Read the model definition and answer for the solid it produces. Units are mm, in the model's axes. A direction names the side the tool comes from. Coordinates: 2 decimals unless noted, no trailing zeros. Loops run counter-clockwise (first coordinate to the right, second up) from the corner with the lowest first, then second, coordinate; pieces in that order, holes last. Notation, with made-up numbers: M 49,42 L 75,42 A27 cw 75,61 Z; hole C -1,-13 d8. An arc over 180 degrees is marked long. One line per item, written item: value. Start each with the question number.
```python
from build123d import *

# Parameters (mm, degrees)
SKETCH_1_R      = 1.25
EXTRUDE_1_DEPTH = 1.6


with BuildPart() as part:
    # Эскиз1 → Бобышка-Вытянуть1 (new body)
    with BuildSketch(Plane(origin=(0, 0, 0), x_dir=(0, 0, -1), z_dir=(1, 0, 0))):
        with BuildLine():
            Line((2.714158993, 32.8544628), (3.027276679, 29.368497035))
            Line((3.027276679, 29.368497035), (-8.924605944, 28.294950683))
            Line((-8.924605944, 28.294950683), (-9.23772363, 31.780916448))
            ThreePointArc((-9.23772363, 31.780916448), (-9.009264175, 32.511390756), (-8.331195608, 32.866368862))
            Line((-8.331195608, 32.866368862), (-4.596232288, 33.201852097))
            Line((-4.596232288, 33.201852097), (-4.417307896, 31.20987166))
            ThreePointArc((-4.417307896, 31.20987166), (-3.991334168, 30.39618938), (-3.114764999, 30.122038033))
            Line((-3.114764999, 30.122038033), (-3.015165977, 30.130984253))
            ThreePointArc((-3.015165977, 30.130984253), (-2.201483696, 30.55695798), (-1.92733235, 31.43352715))
            Line((-1.92733235, 31.43352715), (-2.106256742, 33.425507587))
            Line((-2.106256742, 33.425507587), (1.628706578, 33.760990822))
            ThreePointArc((1.628706578, 33.760990822), (2.359180886, 33.532531367), (2.714158993, 32.8544628))
        make_face()
        with Locations((-6.635920339, 30.759584164)):
            Circle(SKETCH_1_R, mode=Mode.SUBTRACT)
        with Locations((0.336011191, 31.385819536)):
            Circle(SKETCH_1_R, mode=Mode.SUBTRACT)
    extrude(amount=EXTRUDE_1_DEPTH)


solid = part.part
```
1) Section C-C (y = 32.2) is taken. Determine the outline of the cut face in (x, z).
2) Section B-B (z = 0.25) is taken. Determine the outline of the cut face in (x, y), then the cut area to 3 significant figures.
3) Section A-A (y = 33.05) is taken. Determine the outline of the cut face in (x, z), then the cut area to 3 significant figures.
4) A flat-ended cylindrical pin translates along its axis: pin 1 (1.5 mm diameter, centred on y = 31.39, z = -0.34, fed in from +X). Find the tip coordinate at first contact, or state that the pin passes through.
5) A tool of negligible diameter and unlimited length cuts with its end or side. For faces 1 (the face through (0.789, 32.416, 2.016)), 2 (the face through (0.79, 32.22, 4.51)), 3 (the face through (0, 29.9, 3)), from which of +Z, -Z, +X, -X, +Y, -Y can it reach the whole face along a straight path? Write none if from no direction.
6) For a pull along Y with two mould halves and no side action, classify faces 4 (the face through (0.79, 28.84, 2.87)), 5 (the face through (0.789, 30.405, 4.001)), 6 (the face through (0.789, 30.547, 2.21)) as released by +Y, released by -Y, zero draft, split by the parting line, or undercut.
7) Section D-D (y = 30.25) is taken. Determine the outline of the cut face in (x, z), then the cut area to 3 significant figures.
8) Consider line 1 along Z through (x, y) = (0.7, 31.7); line 2 along Z through (x, y) = (1.05, 32.15); line 3 along Z through (x, y) = (1.5, 32.05). Determine where each line is inside the solid, lowest interval first.
Results found:
1. outline: M 0,-2.77 L 1.6,-2.77 L 1.6,-1.28 L 0,-1.28 Z; M 0,0.61 L 1.6,0.61 L 1.6,2 L 0,2 Z; M 0,4.51 L 1.6,4.51 L 1.6,9.19 L 0,9.19 Z
2. outline: M 0,29.07 L 1.6,29.07 L 1.6,30.28 L 0,30.28 Z; M 0,32.49 L 1.6,32.49 L 1.6,33.59 L 0,33.59 Z
2. area: 3.70 mm²
3. outline: M 0,-2.68 L 1.6,-2.68 L 1.6,2.07 L 0,2.07 Z; M 0,4.58 L 1.6,4.58 L 1.6,6.29 L 0,6.29 Z
3. area: 10.3 mm²
4. pin 1: passes through
5. face 1: +X, -X
5. face 2: +X, -X, +Y
5. face 3: +Z, -Z, -X, +Y, -Y
6. face 4: released by -Y
6. face 5: released by +Y
6. face 6: undercut
7. outline: M 0,-2.95 L 1.6,-2.95 L 1.6,-0.86 L 0,-0.86 Z; M 0,0.19 L 1.6,0.19 L 1.6,2.59 L 0,2.59 Z; M 0,3.77 L 1.6,3.77 L 1.6,5.49 L 0,5.49 Z; M 0,7.78 L 1.6,7.78 L 1.6,9.1 L 0,9.1 Z
7. area: 12.1 mm²
8. line 1: z = -2.82 to -1.55, 0.87 to 1.95, 4.46 to 5.81, 7.46 to 9.23
8. line 2: z = -2.78 to -1.33, 0.65 to 1.99, 4.5 to 9.2
8. line 3: z = -2.79 to -1.39, 0.72 to 1.98, 4.49 to 9.23
